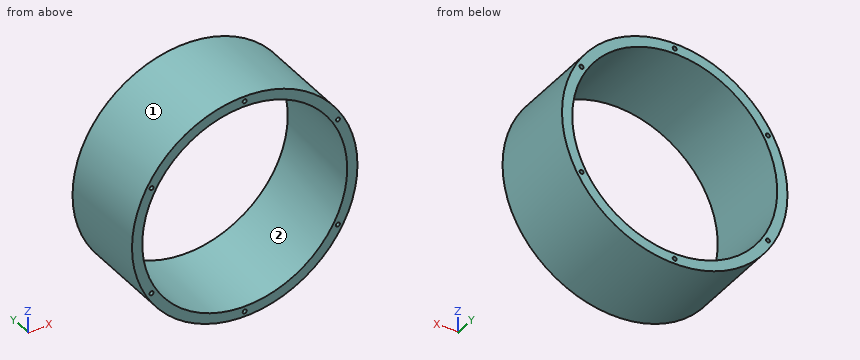
```python
from build123d import *

# Parameters (mm, degrees)
SKETCH1_R         = 69.85
SKETCH1_R_2       = 63.5
EXTRUDE1_DEPTH    = 57.15
CIRPATTERN1_COUNT = 6
CIRPATTERN2_COUNT = 6


with BuildPart() as part:
    # Sketch1 → Extrude1 (new body)
    with BuildSketch(Plane(origin=(0, 0, 0), x_dir=(1, 0, 0), z_dir=(0, 1, 0))):
        Circle(SKETCH1_R)
        Circle(SKETCH1_R_2, mode=Mode.SUBTRACT)
    extrude(amount=EXTRUDE1_DEPTH)

    # Sketch5 → 3-56 Tapped Hole1 (revolve, cut)
    with BuildSketch(Plane(origin=(0, 0, 66.675), x_dir=(0, 0, -1), z_dir=(1, 0, 0))):
        Polygon((0, 0), (0, 6.975736249), (1.0414, 6.35), (1.0414, 5.08), (1.2573, 5.08), (1.2573, 0), align=None)
    f_3_56_tapped_hole1 = revolve(axis=Axis((0, -6.35, 66.675), (0, 1, 0)), mode=Mode.SUBTRACT)

    # CirPattern1: 3-56 Tapped Hole1 ×6 about axis
    cirpattern1_axis = Axis((0, 0, 0), (0, 1, 0))
    for i in range(1, CIRPATTERN1_COUNT):
        add(f_3_56_tapped_hole1.rotate(cirpattern1_axis, i * 360 / CIRPATTERN1_COUNT), mode=Mode.SUBTRACT)

    # Sketch6 → 3-56 Tapped Hole2 (revolve, cut)
    with BuildSketch(Plane(origin=(0.005576043, 57.15, -66.674999767), x_dir=(0, 0, 1), z_dir=(1, 0, 0))):
        Polygon((0, 0), (0, 7.026536249), (1.0414, 6.4008), (1.0414, 5.0292), (1.2573, 5.0292), (1.2573, 0), align=None)
    f_3_56_tapped_hole2 = revolve(axis=Axis((0.005576043, 63.5, -66.674999767), (0, -1, 0)), mode=Mode.SUBTRACT)

    # CirPattern2: 3-56 Tapped Hole2 ×6 about axis
    cirpattern2_axis = Axis((0, 0, 0), (0, 1, 0))
    for i in range(1, CIRPATTERN2_COUNT):
        add(f_3_56_tapped_hole2.rotate(cirpattern2_axis, i * 360 / CIRPATTERN2_COUNT), mode=Mode.SUBTRACT)


solid = part.part
```
Geometry: final body of the model. Coordinates: model frame, mm. Face numbers are marked on the shaded views. Round coordinates to 2 decimals unless told otherwise and drop trailing zeros. Loops run counter-clockwise (first coordinate to the right, second up) from the corner with the lowest first, then second, coordinate; pieces in that order, holes last.
Item 1: Line query: L1, parallel to Z at x = -1, y = 22; L2, parallel to X at y = 50.5, z = 48; L3, parallel to X at y = 53, z = 30. Output: solid intervals per line, ascending.
Checked values:
L1: z = -69.84 to -63.49, 63.49 to 69.84
L2: x = -50.74 to -41.57, 41.57 to 50.74
L3: x = -63.08 to -55.97, 55.97 to 63.08
Item 2: Contact query for flat-ended pins moving along their axis: P1, Ø1, axis at x = 32, y = 28.5, coming from the -Z side; P2, Ø5, axis at y = 41, z = 7.5, coming from the -X side; P3, Ø5, axis at y = 33, z = -23, coming from the +X side. Output: stop coordinate, or through.
Checked values:
P1: stops at z = -62.34
P2: stops at x = -69.67
P3: stops at x = 66.77
Item 3: Mould query, pull axis Z, two halves, no side actions, for the marked faces 1 and 2. Classes: released by +Z, released by -Z, zero draft, split by the parting line, or undercut.
Checked values:
face 1: split by the parting line
face 2: undercut
Item 4: Section C-C, the plane y = 38.5. Output: boundary loops of the cut face in (x, z), plus the area to 3 significant figures.
Checked values:
outline: circle Ø139.7 at (0, 0); hole circle Ø127 at (0, 0)
area: 2,660 mm2
Item 5: Section A-A, the plane z = 0. Output: boundary loops of the cut face in (x, y).
Checked values:
outline: (-69.85, 0) - (-63.5, 0) - (-63.5, 57.15) - (-69.85, 57.15) - close; (63.5, 0) - (69.85, 0) - (69.85, 57.15) - (63.5, 57.15) - close
Item 6: Section B-B, the plane x = 54. Output: boundary loops of the cut face in (y, z), plus the area to 3 significant figures.
Checked values:
outline: (0, -44.31) - (57.15, -44.31) - (57.15, -33.41) - (0, -33.41) - close; (0, 33.41) - (57.15, 33.41) - (57.15, 44.31) - (0, 44.31) - close
area: 1,250 mm2
